```python
from build123d import *

# Parameters (mm, degrees)
F3_DEPTH = 88.138


with BuildPart() as f1:
    # F0 (on Right) → F1 (revolve)
    with BuildSketch(Plane.YZ):
        with BuildLine():
            Line((0, 70.8416298213), (0, -70.8416298213))
            ThreePointArc((0, -70.8416298213), (70.8416298213, 0), (0, 70.8416298213))
        make_face()
    revolve(axis=Axis((0, 0, 0), (0, 0, -1)))

    # F2 (on Front) → F3 (intersect, symmetric)
    with BuildSketch(Plane.XZ):
        with BuildLine():
            add(Edge.make_bspline(
                [(-46.6592088342, 53.2616898417), (-45.4183797693, 54.5278978273), (-42.6869236647, 57.3152209406), (-36.2931747251, 62.1716157185), (-26.9719798216, 65.8489474918), (-18.3180072339, 67.9057468895), (-6.7062624568, 69.3009329626), (4.4643194234, 70.0168470256), (16.9701926515, 67.2645644417), (27.1342814823, 65.9736427336), (38.7911737808, 59.4801067729), (43.6075364693, 55.6569433468), (45.7895621657, 53.9248809218)],
                knots=[0, 0, 0, 0, 0.0747817838, 0.1646182908, 0.2647754033, 0.36017978, 0.4679768944, 0.5753520805, 0.6877157242, 0.7905193986, 0.9050960061, 1, 1, 1, 1], degree=3))
            Line((-46.6592088342, 53.2616898417), (-55.1035441458, 14.7579303011))
            Line((-55.1035441458, 14.7579303011), (-55.1035441458, 12.6094166189))
            Line((-55.1035441458, 12.6094166189), (-57.4055202305, 10.0005073473))
            Line((-57.4055202305, 10.0005073473), (-57.4055202305, -29.4290501624))
            Line((-57.4055202305, -29.4290501624), (-55.1035441458, -31.6015295684))
            Line((-55.1035441458, -31.6015295684), (-51.1359348893, -49.1747111082))
            add(Edge.make_bspline(
                [(-51.1359348893, -49.1747111082), (-47.9992454957, -52.1301607476), (-40.7561015524, -58.9547915828), (-19.1287563078, -69.9086773355), (4.1850416995, -72.4466384159), (27.1525670282, -67.080206471), (42.7802476894, -55.4128974746), (51.1359348893, -49.1747111082)],
                knots=[0, 0, 0, 0, 0.15742802, 0.3635278048, 0.5674104782, 0.7687063865, 1, 1, 1, 1], degree=3))
            Line((51.1359348893, -49.1747111082), (55.1035441458, -31.6015295684))
            Line((55.1035441458, -31.6015295684), (57.4055202305, -29.4290501624))
            Line((57.4055202305, -29.4290501624), (57.4055202305, 10.0005073473))
            Line((57.4055202305, 10.0005073473), (55.1035441458, 14.7579303011))
            Line((55.1035441458, 14.7579303011), (46.6592088342, 53.2616898417))
            Line((46.6592088342, 53.2616898417), (45.7895621657, 53.9248809218))
        make_face()
    extrude(amount=F3_DEPTH, both=True, mode=Mode.INTERSECT)


solid = f1.part
```
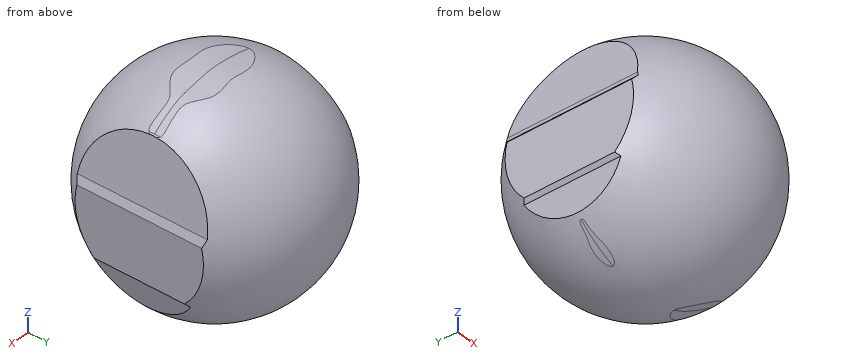
The listing builds one solid part. Answer for the finished solid, in the listing's coordinates (mm). Round coordinates to 2 decimals unless told otherwise and drop trailing zeros. Order: outer loops, then holes, each group sorted by start corner. A loop starts at its lowest first (then second) coordinate and runs counter-clockwise, first axis right, second up. Notation, with made-up numbers: (64, 14) -> (77, 14) arc R20 ccw to (77, 29) -> close; hole circle Ø3 at (58.25, 43.5). An arc over 180 degrees is marked (long way). Answer as CSV lines item,"result". Start each with the question number.
(1) The part is cut by section A-A (y = -21). Determine the outline of the cut face in (x, z).
(2) Flat-ended cylindrical pins translate along their axes: pin 1 Ø1.5 at (x, y) = (-26, 38) entering from +Z; pin 2 Ø1.5 at (y, z) = (11, 31.5) entering from -X; pin 3 Ø1 at (x, z) = (-31, -6.5) entering from -Y. Find the tip coordinate at first contact, or state that the pin passes through.
(3) Find the intervals of material crossed by probe 1 along Y at (x, z) = (-16, -24); probe 2 along X at (y, z) = (-10, 44.5); probe 3 along Z at (x, y) = (15.5, -55.5), in increasing order. Write a range as from..to.
(4) The part is cut by section B-B (z = -20.5). Determine the outline of the cut face in (x, y).
(5) The part is cut by section C-C (z = -4.5). Determine the outline of the cut face in (x, y), then the cut area to 3 significant figures.
Evaluation:
1,outline,"(-57.41, -29.43) -> (-55.1, -31.6) -> (-52.64, -42.5) arc R67.66 ccw to (52.64, -42.5) -> (55.1, -31.6) -> (57.41, -29.43) -> (57.41, 10) -> (55.1, 14.76) -> (47.85, 47.83) arc R67.66 ccw to (-47.85, 47.83) -> (-55.1, 14.76) -> (-55.1, 12.61) -> (-57.41, 10) -> close"
2,pin 1,"z = 54.47"
2,pin 2,"x = -51.6"
2,pin 3,"y = -63.61"
3,probe 1,"-64.7..64.7"
3,probe 2,"-48.58..48.58"
3,probe 3,"-41.21..41.21"
4,outline,"(-57.41, -36.1) arc R67.81 ccw to (57.41, -36.1) -> (57.41, 36.1) arc R67.81 ccw to (-57.41, 36.1) -> close"
5,outline,"(-57.41, -41.27) arc R70.7 ccw to (57.41, -41.27) -> (57.41, 41.27) arc R70.7 ccw to (-57.41, 41.27) -> close"
5,area,"14,200 mm²"
